Part print with two shaded views. Sizes in mm from the minimum x, y, z corner. A direction names the side the tool comes from. Round coordinates to 2 decimals unless told otherwise and drop trailing zeros. Write each loop counter-clockwise with the first axis right and the second up, starting at its lowest first coordinate (ties: lowest second). Pieces come first, ordered by that corner, then holes. Notation, with made-up numbers: (-23, 84) -> (6, 84) arc R25 cw to (6, 101) -> close; hole circle Ø8 at (75, 16). An arc over 180 degrees is marked (long way). Return JSON: item names as keys, results as strings. Group by question number.
(1) Saw through at C-C (x = 16). List the corners of the cut face in (y, z) (1 decimal), plus the area to 3 significant figures.
(2) Mould opens along Z. For the marked faces 1, 2 and 3 say: +Z half, -Z half, draft (parallel to the pull), parting line (faces both ways), or undercut.
(3) Saw through at A-A (y = 12.7). List the corners of the cut face in (x, z) (1 decimal).
(4) Drill centre lines: L1, parallel to X at y = 2, z = 12.7; L2, parallel to Z at x = 6.5, y = 19.25 (1 decimal). Where is each one in solid material? Low to high. Write a range as from..to.
(5) Drop flat-ended pins along their axis: pin 1 Ø5 at (x, z) = (20, 5) entering from +Y; pin 2 Ø9 at (x, z) = (17.46, 12.7) entering from +Y (1 decimal); pin 3 Ø10 at (x, y) = (14.5, 10) entering from +Z (1 decimal). Give the stop position or say it passes through.
(6) Tool access for the marked faces 4 and 5: list every direction of +Z, -Z, +X, -X, +Y, -Y with a clear straight run to the whole face (end or side of a thin tool).
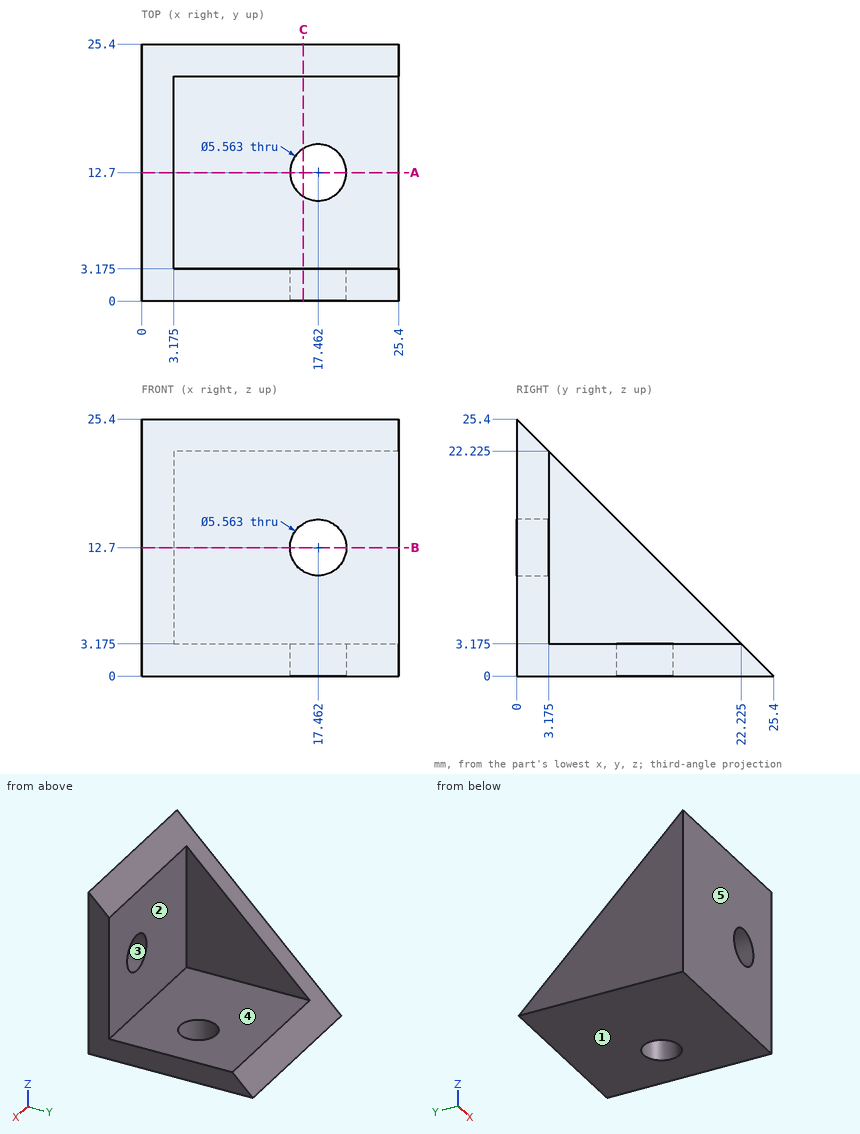
Computed values:
{
 "1": {"outline": "(0, 0) -> (10.3, 0) -> (10.3, 3.2) -> (3.2, 3.2) -> (3.2, 10.3) -> (0, 10.3) -> close; (0, 15.1) -> (3.2, 15.1) -> (3.2, 22.2) -> (0, 25.4) -> close; (15.1, 0) -> (25.4, 0) -> (22.2, 3.2) -> (15.1, 3.2) -> close", "area": "111 mm2"},
 "2": {"face 1": "-Z half", "face 2": "draft", "face 3": "undercut"},
 "3": {"outline": "(0, 0) -> (14.7, 0) -> (14.7, 3.2) -> (3.2, 3.2) -> (3.2, 12.7) -> (0, 12.7) -> close; (20.2, 0) -> (25.4, 0) -> (25.4, 3.2) -> (20.2, 3.2) -> close"},
 "4": {"L1": "0..14.68, 20.24..25.4", "L2": "0..3.2"},
 "5": {"pin 1": "y = 22.9", "pin 2": "y = 3.2", "pin 3": "z = 3.2"},
 "6": {"face 4": "+Z, +X, +Y", "face 5": "+Z, -Z, +X, -X, -Y"}
}
